Build history of the part. All positions in model axes, mm. Face numbers are marked on the shaded views. A direction names the side the tool comes from. Give positions to 0.01 mm unless a question says otherwise; leave off trailing zeros. Write each loop counter-clockwise with the first axis right and the second up, starting at its lowest first coordinate (ties: lowest second). Pieces come first, ordered by that corner, then holes.
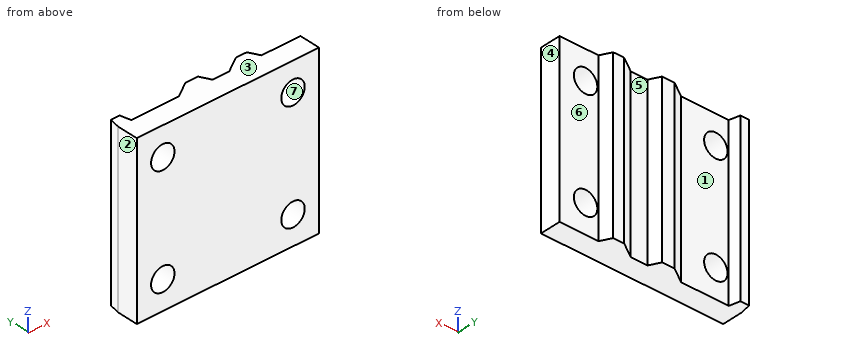
from build123d import *

# Parameters (mm, degrees)
SKETCH_1_W      = 35
SKETCH_1_H      = 32
SKETCH_1_R      = 2.25
EXTRUDE_1_DEPTH = 4
EXTRUDE_2_DEPTH = 32


with BuildPart() as part:
    # 草图1 → 凸台-拉伸1 (new body)
    with BuildSketch(Plane(origin=(0, 0, 0), x_dir=(1, 0, 0), z_dir=(0, 1, 0))):
        Rectangle(SKETCH_1_W, SKETCH_1_H)
        with Locations(Location((-12.5, 10.5, 0), (0, 0, 270))):
            Circle(SKETCH_1_R, mode=Mode.SUBTRACT)
        with Locations(Location((-12.5, -10.5, 0), (0, 0, 90))):
            Circle(SKETCH_1_R, mode=Mode.SUBTRACT)
        with Locations(Location((12.5, -10.5, 0), (0, 0, 270))):
            Circle(SKETCH_1_R, mode=Mode.SUBTRACT)
        with Locations(Location((12.5, 10.5, 0), (0, 0, 90))):
            Circle(SKETCH_1_R, mode=Mode.SUBTRACT)
    extrude(amount=EXTRUDE_1_DEPTH)

    # 草图3 → 凸台-拉伸2 (add)
    with BuildSketch(Plane.XY.offset(16)):
        Polygon((6.872858809, 6), (3.83657923, 4), (10.023141572, 4), (8.981867617, 6), align=None)
        Polygon((-2.800937358, 6), (-5.837216937, 4), (0.634129455, 4), (-0.4071445, 6), align=None)
        Polygon((-17.09182921, 6), (-17.5, 4), (-14.975210984, 4), (-15.433336788, 6), align=None)
    extrude(amount=-EXTRUDE_2_DEPTH)


solid = part.part
(1) 3-axis set-ups, long thin cutter, end or side, ignore diameter. For the marked faces 5, 6 and 7: which of +Z, -Z, +X, -X, +Y, -Y reach the whole face in a straight line?
(2) Saw through at B-B, the plane x = -12.5. List the corners of the cut face in (y, z), plus the area to 3 significant figures.
(3) Probe line 1 (X direction, y = 0.8, z = 10.5); line 2 (X direction, y = 2.3, z = -12); line 3 (Z direction, x = 14, y = 2.35). List the from-to ranges inside material, lowest first.
(4) Saw through at D-D, the plane z = -1. List the corners of the cut face in (x, y).
(5) Mould opens along X. For the marked faces 1, 2, 3 and 4 say: +X half, -X half, draft (parallel to the pull), parting line (faces both ways), or undercut.
(6) Saw through at A-A, the plane z = -10.5. List the corners of the cut face in (x, y), plus the area to 3 significant figures.
(7) Drop flat-ended pins along their axis: pin 1 (2.5 mm diameter, centred on x = -12.5, z = 1.5, fed in from +Y); pin 2 (8 mm diameter, centred on x = -7, z = -12, fed in from -Y); pin 3 (6 mm diameter, centred on x = 12.5, z = -10.5, fed in from +Y); pin 4 (3.5 mm diameter, centred on x = 3, z = -5, fed in from +Y). Give the stop position or say it passes through.
(8) Saw through at C-C, the plane y = 4.9. List the corners of the cut face in (x, z).
Computed values:
1. face 5: +Z, -Z, +Y
1. face 6: +Z, -Z, +X, +Y
1. face 7: +Y, -Y
2. outline: (0, -16) - (4, -16) - (4, -12.75) - (0, -12.75) - close; (0, -8.25) - (4, -8.25) - (4, 8.25) - (0, 8.25) - close; (0, 12.75) - (4, 12.75) - (4, 16) - (0, 16) - close
2. area: 92.0 mm2
3. line 1: x = -17.5 to -14.75, -10.25 to 10.25, 14.75 to 17.5
3. line 2: x = -17.5 to -14.18, -10.82 to 10.82, 14.18 to 17.5
3. line 3: z = -16 to -12.18, -8.82 to 8.82, 12.18 to 16
4. outline: (-17.5, 0) - (17.5, 0) - (17.5, 4) - (10.02, 4) - (8.98, 6) - (6.87, 6) - (3.84, 4) - (0.63, 4) - (-0.41, 6) - (-2.8, 6) - (-5.84, 4) - (-14.98, 4) - (-15.43, 6) - (-17.09, 6) - (-17.5, 4) - close
5. face 1: undercut
5. face 2: -X half
5. face 3: draft
5. face 4: +X half
6. outline: (-17.5, 0) - (-14.75, 0) - (-14.75, 4) - (-14.98, 4) - (-15.43, 6) - (-17.09, 6) - (-17.5, 4) - close; (-10.25, 0) - (10.25, 0) - (10.25, 4) - (10.02, 4) - (8.98, 6) - (6.87, 6) - (3.84, 4) - (0.63, 4) - (-0.41, 6) - (-2.8, 6) - (-5.84, 4) - (-10.25, 4) - close; (14.75, 0) - (17.5, 0) - (17.5, 4) - (14.75, 4) - close
6. area: 125 mm2
7. pin 1: stops at y = 4
7. pin 2: stops at y = 0
7. pin 3: stops at y = 5
7. pin 4: stops at y = 4.6
8. outline: (-17.32, -16) - (-15.18, -16) - (-15.18, 16) - (-17.32, 16) - close; (-4.47, -16) - (0.17, -16) - (0.17, 16) - (-4.47, 16) - close; (5.2, -16) - (9.55, -16) - (9.55, 16) - (5.2, 16) - close
